```python
from build123d import *

# Parameters (mm, degrees)
F6_DEPTH = 15
F8_D     = 8.5


with BuildPart() as f2:
    # F0 (on Front) → F2 (revolve)
    with BuildSketch(Plane.XZ):
        with BuildLine():
            Line((-15, 0), (15, 0))
            ThreePointArc((15, 0), (3.8822856765, 14.4888873943), (-12.9903810568, 7.5))
            ThreePointArc((-12.9903810568, 7.5), (-14.4888873943, 3.8822856765), (-15, 0))
        make_face()
        with BuildLine():
            ThreePointArc((-15, 0), (-14.4888873943, 3.8822856765), (-12.9903810568, 7.5))
            Line((-12.9903810568, 7.5), (-37.3508893593, 6))
            ThreePointArc((-37.3508893593, 6), (-36.3418971125, 3.0750976432), (-36, 0))
            Line((-36, 0), (-15, 0))
        make_face()
    revolve(axis=Axis((-10.5, 0, 0), (-1, 0, 0)))

    # F0 (on Front) → F3 (revolve)
    with BuildSketch(Plane.XZ):
        with BuildLine():
            ThreePointArc((-36, 0), (-36.3418971125, 3.0750976432), (-37.3508893593, 6))
            ThreePointArc((-37.3508893593, 6), (-39.3230376655, 9.0555218131), (-42.0156402887, 11.5))
            Line((-42.0156402887, 11.5), (-50, 11.5))
            Line((-50, 11.5), (-50, -9.5))
            Line((-50, -9.5), (-39.7165180994, -9.5))
            ThreePointArc((-39.7165180994, -9.5), (-38.4009289093, -7.8397416943), (-37.3508893593, -6))
            ThreePointArc((-37.3508893593, -6), (-36.3418971125, -3.0750976432), (-36, 0))
        make_face()
    revolve(axis=Axis((-50, 0, 1), (0, 0, 1)))

    # F0 (on Front) → F4 (revolve)
    with BuildSketch(Plane.XZ):
        with BuildLine():
            ThreePointArc((-64, 0), (-63.7672392953, 2.542267135), (-63.0766968306, 5))
            Line((-63.0766968306, 5), (-89.0912878854, 5))
            ThreePointArc((-89.0912878854, 5), (-88.2759958765, 2.5588527336), (-88, 0))
            Line((-88, 0), (-64, 0))
        make_face()
    revolve(axis=Axis((-76, 0, 0), (1, 0, 0)))

    # F0 (on Front) → F5 (revolve)
    with BuildSketch(Plane.XZ):
        with BuildLine():
            ThreePointArc((-88, 0), (-88.2759958765, 2.5588527336), (-89.0912878854, 5))
            ThreePointArc((-89.0912878854, 5), (-90.0598209908, 6.7225621057), (-91.2979315152, 8.2628084866))
            Line((-91.2979315152, 8.2628084866), (-100, 8.2628084866))
            Line((-100, 8.2628084866), (-100, -12))
            ThreePointArc((-100, -12), (-93.5192593016, -10.0995049384), (-89.0912878854, -5))
            ThreePointArc((-89.0912878854, -5), (-88.2759958765, -2.5588527336), (-88, 0))
        make_face()
    revolve(axis=Axis((-100, 0, -1.8685957567), (0, 0, -1)))

    # F1 (on Top) → F6 (cut, symmetric)
    with BuildSketch(Plane.XY):
        with BuildLine():
            Line((-41.6, 1.5), (-43.1626028344, 1.5))
            ThreePointArc((-43.1626028344, 1.5), (-57, 0), (-43.1626028344, -1.5))
            Line((-43.1626028344, -1.5), (-41.6, -1.5))
            Line((-41.6, -1.5), (-41.6, 1.5))
        make_face()
    extrude(amount=F6_DEPTH, both=True, mode=Mode.SUBTRACT)

    # F8 (through all)
    with Locations(Plane.XY.offset(8.2628084866)):
        with Locations((-100, 0)):
            Hole(F8_D / 2)


solid = f2.part
```
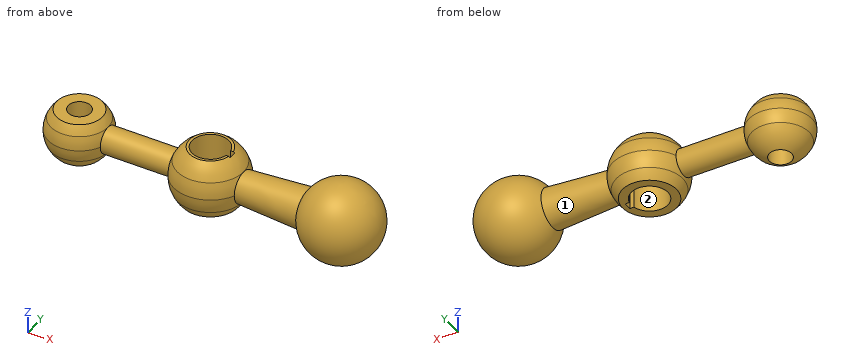
Part model, mm, in its own coordinate system. Face numbers are marked on the shaded views. A direction names the side the tool comes from. Round coordinates to 2 decimals unless told otherwise and drop trailing zeros. Loops run counter-clockwise (first coordinate to the right, second up) from the corner with the lowest first, then second, coordinate; pieces in that order, holes last.
Item 1: Cut at C-C, the plane x = -100. Give the cut face in (y, z).
Item 2: Drill centre lines: line 1 (X direction, y = 0, z = 0); line 2 (X direction, y = 0, z = -3.25); line 3 (Y direction, x = -50, z = -3.75). Where is each one in solid material? Low to high.
Item 3: 3-axis set-ups, long thin cutter, end or side, ignore diameter. For the marked faces 1 and 2: which of +Z, -Z, +X, -X, +Y, -Y reach the whole face in a straight line?
Item 4: Cut at A-A, the plane x = -50. Give the cut face in (y, z), then the cut area to 3 significant figures.
Item 5: Cut at B-B, the plane y = 0. Give the cut face in (x, z), then the cut area to 3 significant figures.
Item 6: Drop flat-ended pins along their axis: P1, Ø5, axis at x = -100, y = 0, coming from the -Z side; P2, Ø1.7, axis at x = -42, z = 1, coming from the +Y side; P3, Ø6, axis at x = -52, y = 4, coming from the -Z side; P4, Ø1.5, axis at x = -1, z = -0.5, coming from the +Y side. Give the stop position or say it passes through.
Item 7: Cut at D-D, the plane x = -9. Give the cut face in (y, z).
A:
1. outline: (-8.7, 8.26) arc R12 ccw to (-4.25, -11.22) - (-4.25, 8.26) - close; (4.25, -11.22) arc R12 ccw to (8.7, 8.26) - (4.25, 8.26) - close
2. line 1: x = -112 to -104.25, -95.75 to -57, -41.6 to 15
2. line 2: x = -111.55 to -104.25, -95.75 to -57, -41.6 to 14.64
2. line 3: y = -13.49 to -7, 7 to 13.49
3. face 1: none
3. face 2: +Z, -Z
4. outline: (-10.28, -9.5) - (-7, -9.5) - (-7, 11.5) - (-7.98, 11.5) arc R14 ccw to start; (7, -9.5) - (10.28, -9.5) arc R14 ccw to (7.98, 11.5) - (7, 11.5) - close
4. area: 231 mm2
5. outline: (-108.7, 8.26) arc R12 ccw to (-104.25, -11.22) - (-104.25, 8.26) - close; (-95.75, -11.22) arc R12 ccw to (-89.09, -5) - (-63.08, -5) arc R14 ccw to (-60.28, -9.5) - (-57, -9.5) - (-57, 11.5) - (-57.98, 11.5) arc R14 ccw to (-63.08, 5) - (-89.09, 5) arc R12 ccw to (-91.3, 8.26) - (-95.75, 8.26) - close; (-41.6, -9.5) - (-39.72, -9.5) arc R14 ccw to (-37.35, -6) - (-12.99, -7.5) arc R15 ccw (long way) to (-12.99, 7.5) - (-37.35, 6) arc R14 ccw to (-41.6, 11.2) - close
5. area: 1,690 mm2
6. P1: passes through
6. P2: stops at y = 12
6. P3: stops at z = -9.5
6. P4: stops at y = 15
7. outline: circle Ø24 at (0, 0)
